Autodesk Inventor part; units mm, degrees
ref_plane "YZ Plane" through (0, 0, 0) normal (1, 0, 0) x (0, 1, 0)
ref_plane "XZ Plane" through (0, 0, 0) normal (0, 1, 0) x (-1, 0, 0)
ref_plane "XY Plane" through (0, 0, 0) normal (0, 0, 1) x (1, 0, 0)
sketch "Szkic1" plane through (0, 0, 0) normal (0, 0, 1) x (1, 0, 0)
  line L0 (0, 12.1176) -> (0, -2.0196) construction
  line L1 (-9.6, 0) -> (1.6, 0) construction
  line L2 (0, 0) -> (-8, 0)
  line L3 (-8, 0) -> (-8, 6.098)
  line L4 (-8, 6.098) -> (0, 6.098)
  line L5 (0, 6.098) -> (0, 0)
  circle A0 centre (-4, 6.098) radius 4
  dimension "d0" = 8
  dimension "d1" = 6.098
extrude "Wyciągnięcie proste1" add sketch "Szkic1" along normal blind 2
hole "Otwór1" at (-4, 6.098, 0) direction (0, 0, 1) diameter 2 end through all
fillet "Zaokrąglenie1" radius 2 3 edges at (-4, 10.098, 2) (-8, 3.049, 2) (0, 3.049, 2)
properties part number "podpora_kciuk"
Source: CAD feature listing. Evaluate the final solid. Frame: model axes, mm. Round coordinates to 2 decimals unless told otherwise and drop trailing zeros. Loops run counter-clockwise (first coordinate to the right, second up) from the corner with the lowest first, then second, coordinate; pieces in that order, holes last. Notation, with made-up numbers: M -23,19 L 20,19 A25 cw 20,56 Z; hole C 84.5,70.5 d5. An arc over 180 degrees is marked long. Use a Markdown table: item, result. Add a question column.
1. Contact query for flat-ended pins moving along their axis: P1, Ø2, axis at x = -7, y = 2, coming from the +Z side; P2, Ø1, axis at y = 8, z = 1, coming from the +X side; P3, Ø1, axis at y = 8, z = 1, coming from the -X side. Output: stop coordinate, or through.
2. Line query: line 1 (Y direction, x = -4, z = 0.5); line 2 (Y direction, x = -4, z = 1.2); line 3 (X direction, y = 6.5, z = 1.45). Output: solid intervals per line, ascending.
3. Section query C-C on z = 0.6. Return the cut outline in (x, y).
4. Mould query, pull axis Y, two halves, no side actions, for faces 1 (the flat face through (-4, 0, 1)), 2 (the cylindrical face through (-7.4, 3.01, 1.43)), 3 (the cylindrical face through (-4.676, 5.361, 1.014)). Classes: pulls with the +Y half, pulls with the -Y half, needs draft (parallel to the pull), parting line crosses it, or undercut.
5. Section query B-B on z = 1.1. Return the cut outline in (x, y).
Reported:
| question | item | result |
|---|---|---|
| 1 | P1 | stops at z = 2 |
| 1 | P2 | stops at x = -0.43 |
| 1 | P3 | stops at x = -7.57 |
| 2 | line 1 | y = 0 to 5.1, 7.1 to 10.03 |
| 2 | line 2 | y = 0 to 5.1, 7.1 to 9.7 |
| 2 | line 3 | x = -7.35 to -4.92, -3.08 to -0.65 |
| 3 | outline | M -7.91,0 L -0.09,0 L -0.09,6.1 A3.91 ccw -7.91,6.1 Z; hole C -4,6.1 d2 |
| 4 | face 1 | pulls with the -Y half |
| 4 | face 2 | needs draft |
| 4 | face 3 | undercut |
| 5 | outline | M -7.67,0 L -0.33,0 L -0.33,6.1 A3.67 ccw -7.67,6.1 Z; hole C -4,6.1 d2 |
